For this review, take the finished solid that the model builds, in its own axes (mm). A direction names the side the tool comes from. Round coordinates to 2 decimals unless told otherwise and drop trailing zeros. Order: outer loops, then holes, each group sorted by start corner. A loop starts at its lowest first (then second) coordinate and runs counter-clockwise, first axis right, second up. Notation, with made-up numbers: (56, 36) -> (88, 36) arc R29 cw to (88, 70) -> close; hole circle Ø2 at (59.5, 57.25). An arc over 180 degrees is marked (long way). Answer in a Markdown table with one row per item.
```python
from build123d import *

# Parameters (mm, degrees)
SKETCH_1_R          = 3.6
EXTRUDE_1_DEPTH     = 8.8
SKETCH_2_W          = 6
SKETCH_2_H          = 12
EXTRUDE_2_DEPTH     = 30
SKETCH_4_W          = 6
SKETCH_4_H          = 12
EXTRUDE_3_DEPTH     = 30
SKETCH_3_R          = 2
CUT_EXTRUDE_1_DEPTH = 30
SKETCH_5_W          = 6
SKETCH_5_H          = 8.4
CUT_EXTRUDE_2_DEPTH = 28
SKETCH_6_W          = 6
SKETCH_6_H          = 8.4
CUT_EXTRUDE_3_DEPTH = 28


with BuildPart() as part:
    # 草图1 → 凸台-拉伸1 (new body)
    with BuildSketch(Plane.XY):
        Circle(SKETCH_1_R)
    extrude(amount=EXTRUDE_1_DEPTH)

    # 草图2 → 凸台-拉伸2 (add)
    with BuildSketch(Plane.XY.offset(8.8)):
        Rectangle(SKETCH_2_W, SKETCH_2_H)
    extrude(amount=EXTRUDE_2_DEPTH)

    # 草图4 → 凸台-拉伸3 (add)
    with BuildSketch(Plane(origin=(0, 0, 0), x_dir=(-1, 0, 0), z_dir=(0, 0, -1))):
        Rectangle(SKETCH_4_W, SKETCH_4_H)
    extrude(amount=EXTRUDE_3_DEPTH)

    # 草图3 → 切除-拉伸1 (cut)
    with BuildSketch(Plane(origin=(0, 6, 0), x_dir=(1, 0, 0), z_dir=(0, 1, 0))):
        with Locations((0, -35.6)):
            Circle(SKETCH_3_R)
        with Locations((0, 27.2)):
            Circle(SKETCH_3_R)
    extrude(amount=-CUT_EXTRUDE_1_DEPTH, mode=Mode.SUBTRACT)

    # 草图5 → 切除-拉伸2 (cut)
    with BuildSketch(Plane(origin=(0, 0, -30), x_dir=(-1, 0, 0), z_dir=(0, 0, -1))):
        Rectangle(SKETCH_5_W, SKETCH_5_H)
    extrude(amount=-CUT_EXTRUDE_2_DEPTH, mode=Mode.SUBTRACT)

    # 草图6 → 切除-拉伸3 (cut)
    with BuildSketch(Plane.XY.offset(38.8)):
        Rectangle(SKETCH_6_W, SKETCH_6_H)
    extrude(amount=-CUT_EXTRUDE_3_DEPTH, mode=Mode.SUBTRACT)


solid = part.part
```
Q1. Take a section at C-C, the plane x = 0. Give the number of separate pieces and of enclosed holes in the cut face, then the cut area to 3 significant figures.
Answer key:
| item | result |
|---|---|
| separate pieces | 5 |
| enclosed holes | 0 |
| area | 284 mm^2 |
Q2. Clearance check with flat-ended pins moving along their axes: pin 1 Ø1.5 at (x, y) = (2.5, 0.5) entering from +Z; pin 2 Ø0.7 at (x, y) = (-3.5, 0.5) entering from +Z; pin 3 Ø4 at (y, z) = (-4.5, -3.5) entering from -X. State where each tip first meets the part, or that it passes through.
Answer key:
| item | result |
|---|---|
| pin 1 | stops at z = 10.8 |
| pin 2 | stops at z = 8.8 |
| pin 3 | stops at x = -3 |
Q3. Take a section at B-B, the plane z = 35.6. Write out the cut boundary in (x, y).
Answer key:
| item | result |
|---|---|
| outline | (-3, -6) -> (-2, -6) -> (-2, -4.2) -> (-3, -4.2) -> close; (-3, 4.2) -> (-2, 4.2) -> (-2, 6) -> (-3, 6) -> close; (2, -6) -> (3, -6) -> (3, -4.2) -> (2, -4.2) -> close; (2, 4.2) -> (3, 4.2) -> (3, 6) -> (2, 6) -> close |
Q4. The part is to be moulded in two halves that separate along Z. For faces 4 (the face through (0, 6, 24)), 5 (the face through (0.923, -5.087, 37.374)), 6 (the face through (-0.434, -5.087, -25.248)), 7 (the face through (0, 5, -30)), say which applies: +Z half, -Z half, draft (parallel to the pull), parting line (faces both ways), or undercut.
Answer key:
| item | result |
|---|---|
| face 4 | draft |
| face 5 | undercut |
| face 6 | undercut |
| face 7 | -Z half |
Q5. Take a section at D-D, the plane y = 0. Write out the cut boundary in (x, z).
Answer key:
| item | result |
|---|---|
| outline | (-3.6, 0) -> (-3, 0) -> (-3, -2) -> (3, -2) -> (3, 0) -> (3.6, 0) -> (3.6, 8.8) -> (3, 8.8) -> (3, 10.8) -> (-3, 10.8) -> (-3, 8.8) -> (-3.6, 8.8) -> close |
Q6. Take a section at A-A, the plane y = -5. Write out the cut boundary in (x, z), then the cut area to 3 significant figures.
Answer key:
| item | result |
|---|---|
| outline | (-3, -30) -> (3, -30) -> (3, 0) -> (-3, 0) -> close; (-3, 8.8) -> (3, 8.8) -> (3, 38.8) -> (-3, 38.8) -> close; hole circle Ø4 at (0, -27.2); hole circle Ø4 at (0, 35.6) |
| area | 335 mm^2 |
Q7. To check wall thickness, follow probe 1 along Z at (x, y) = (0, 5.3); probe 2 along Y at (x, z) = (2.25, 34); probe 3 along Z at (x, y) = (1.25, 4.75). State the ranges of each line that lie inside material, in increasing order.
Answer key:
| item | result |
|---|---|
| probe 1 | z = -30 to -29.2, -25.2 to 0, 8.8 to 33.6, 37.6 to 38.8 |
| probe 2 | y = -6 to -4.2, 4.2 to 6 |
| probe 3 | z = -30 to -28.76, -25.64 to 0, 8.8 to 34.04, 37.16 to 38.8 |
Q8. Tool access review of faces 1 (the face through (0, -4.2, 25)), 2 (the face through (0, -4.2, -16)), 3 (the face through (3.434, 1.081, 4.338)): name each direction out of +Z, -Z, +X, -X, +Y, -Y from which nothing blocks a thin tool from reaching the whole face with its end or side.
Answer key:
| item | result |
|---|---|
| face 1 | +Z, +X, -X |
| face 2 | -Z, +X, -X |
| face 3 | none |
